For this review, take the finished solid that the model builds, in its own axes (mm). A direction names the side the tool comes from. Coordinates: 2 decimals unless noted, no trailing zeros. Order: outer loops, then holes, each group sorted by start corner. A loop starts at its lowest first (then second) coordinate and runs counter-clockwise, first axis right, second up. Notation, with made-up numbers: M 12.5,39.25 L 42.5,39.25 A18 ccw 42.5,44.25 Z; hole C 55.5,83 d1. An arc over 180 degrees is marked long. Use CSV: the item, a comma, the result in double quotes.
Autodesk Fusion 360 part; units mm, degrees
sketch "Sketch1" plane through (0, 0, 0) normal (0, 1, 0) x (1, 0, 0)
  line L0 (0, 0) -> (40, 0)
  line L1 (40, 0) -> (40, -70)
  line L2 (40, -70) -> (0, -70)
  line L3 (0, -70) -> (0, 0)
  circle A0 centre (20, -15) radius 5
  circle A1 centre (20, -15) radius 11
  circle A2 centre (14.5, -20.5) radius 1.5
  circle A3 centre (25.5, -20.5) radius 1.5
  circle A4 centre (14.5, -9.5) radius 1.5
  circle A5 centre (25.5, -9.5) radius 1.5
  line L4 (20, -20) -> (20, -67) construction
  line L5 (0, -57) -> (40, -57) construction
  line L6 (20, -20) -> (20, -15) construction
  point P0 (20, -15)
  dimension "d1" = 40
  dimension "d2" = 70
  dimension "d3" = 10
  dimension "d4" = 15
  dimension "d5" = 22
  dimension "d6" = 11
  dimension "d7" = 11
  dimension "d8" = 3
  dimension "d9" = 3
  dimension "d10" = 3
  dimension "d11" = 3
  dimension "d12" = 52
  dimension "d13" = 42
extrude "Extrude1" add sketch "Sketch1" along normal blind 25 contours L0 L1 L2 L3 | A1 | A2 | A3 | A4 | A5
extrude "Extrude2" cut sketch "Sketch1" along normal blind 4 contours A1
extrude "Extrude3" cut sketch "Sketch1" along normal blind 27 contours A2 | A3 | A4 | A5
Item 1: To check wall thickness, follow line 1 along X through (y, z) = (13.5, 20.5); line 2 along Z through (x, y) = (14.5, 14.75); line 3 along X through (y, z) = (19.25, 15). State the ranges of each line that lie inside material, in increasing order. Write a range as [from, to].
Solutions:
line 1,"[0, 13], [16, 24], [27, 40]"
line 2,"[0, 8], [11, 19], [22, 70]"
line 3,"[0, 15], [25, 40]"
Item 2: Add section C-C on y = 21. State the section outline as (x, z) points.
Solutions:
outline,"M 0,0 L 40,0 L 40,70 L 0,70 Z; hole C 14.5,9.5 d3; hole C 14.5,20.5 d3; hole C 20,15 d10; hole C 25.5,9.5 d3; hole C 25.5,20.5 d3"
Item 3: Add section A-A on x = 20. State the section outline as (y, z) points, and give its area (3 significant figures).
Solutions:
outline,"M 0,0 L 25,0 L 25,10 L 4,10 L 4,4 L 0,4 Z; M 0,26 L 4,26 L 4,20 L 25,20 L 25,70 L 0,70 Z"
area,"1,450 mm^2"
Item 4: Add section B-B on z = 15. State the section outline as (x, y) points.
Solutions:
outline,"M 0,0 L 9,0 L 9,4 L 15,4 L 15,25 L 0,25 Z; M 25,4 L 31,4 L 31,0 L 40,0 L 40,25 L 25,25 Z"
Item 5: Add section D-D on x = 26. State the section outline as (y, z) points.
Solutions:
outline,"M 0,0 L 25,0 L 25,8.09 L 4,8.09 L 4,5.78 L 0,5.78 Z; M 0,24.22 L 4,24.22 L 4,21.91 L 25,21.91 L 25,70 L 0,70 Z; M 4,10.91 L 25,10.91 L 25,19.09 L 4,19.09 Z"
Item 6: Draft analysis for pull direction X (two halves, no side actions). For faces 3 (the face through (0, 12, 35)), 4 (the face through (25.076, 1.972, 5.241)), 5 (the face through (20, 25, 35)), 6 (the face through (13.39, 14.35, 21.51)), state which applies: released by +X, released by -X, zero draft, split by the parting line, or undercut.
Solutions:
face 3,"released by -X"
face 4,"undercut"
face 5,"zero draft"
face 6,"undercut"
Item 7: For faces 1 (the face through (25, 4, 17)), 2 (the face through (20, 12, 0)), list the 3-axis set-ups (+Z, -Z, +X, -X, +Y, -Y) from which the entire face can be reached by the end or side of a thin tool; tool diameter is ignored.
Solutions:
face 1,"-Y"
face 2,"-Z, +X, -X, +Y, -Y"
Item 8: Clearance check with flat-ended pins moving along their axes: pin 1 Ø8 at (x, y) = (21.5, 6) entering from -Z; pin 2 Ø4 at (x, z) = (14.5, 20.5) entering from -Y. State where each tip first meets the part, or that it passes through.
Solutions:
pin 1,"z = 0"
pin 2,"y = 4"
